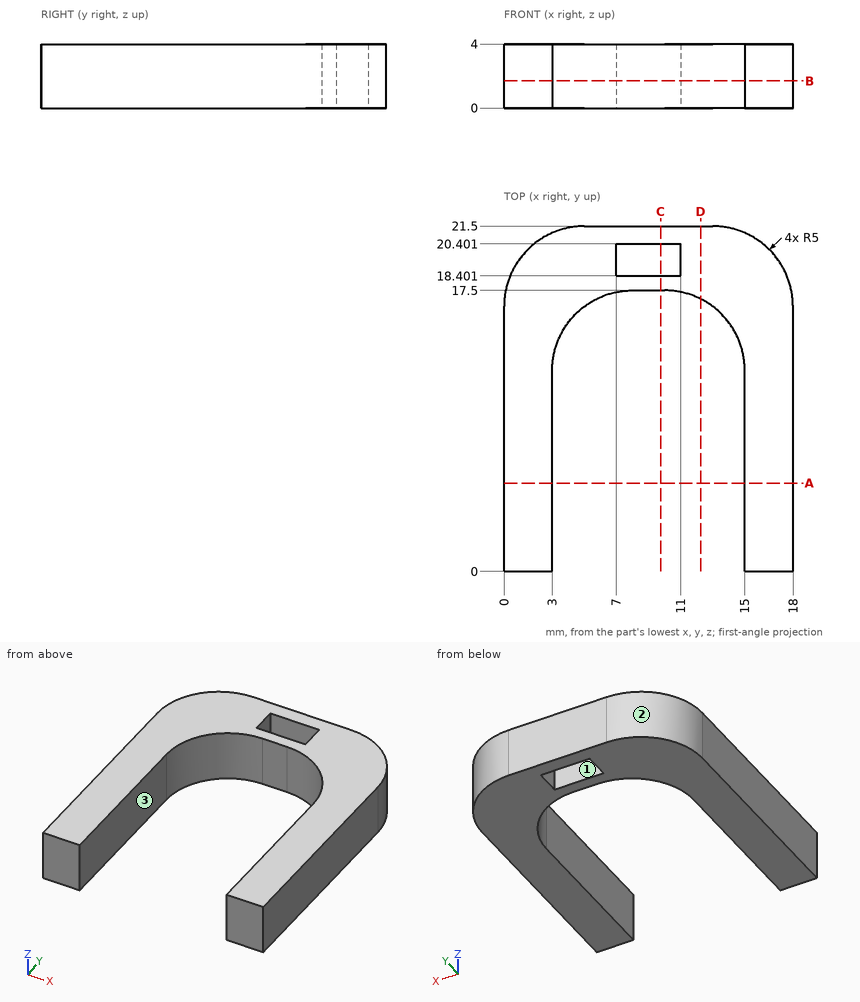
Input: dimensioned drawing with shaded views. Units: mm. Origin: part minimum x, y, z. A direction names the side the tool comes from. Round coordinates to 2 decimals unless told otherwise and drop trailing zeros. Loops run counter-clockwise (first coordinate to the right, second up) from the corner with the lowest first, then second, coordinate; pieces in that order, holes last. Notation, with made-up numbers: M 74.25,-14 L 124.25,-14 A22 ccw 124.25,6 Z; hole C 82,7 d7. An arc over 180 degrees is marked long. Answer in a Markdown table with one row per item. Add a question column.
1. Section B-B (z = 1.7). Output: boundary loops of the cut face in (x, y).
2. Section D-D (x = 12.25). Output: boundary loops of the cut face in (y, z), and give its area (3 significant figures).
3. Section A-A (y = 5.5). Output: boundary loops of the cut face in (x, z), and give its area (3 significant figures).
4. Contact query for flat-ended pins moving along their axis: pin 1 (0.6 mm diameter, centred on x = 9, z = 3, fed in from -Y); pin 2 (0.6 mm diameter, centred on y = 19.5, z = 1.5, fed in from +X); pin 3 (1 mm diameter, centred on y = 19, z = 2, fed in from -X). Output: stop coordinate, or through.
5. Ray query, probe 1 along X at (y, z) = (6.5, 1.85); probe 2 along Y at (x, z) = (9, 1.6); probe 3 along Y at (x, z) = (6, 3.3). Return the intervals inside material, ascending.
6. Set-up query: the marked faces 1, 2 and 3. Return all of +Z, -Z, +X, -X, +Y, -Y with unobstructed straight access to the full face (end or side cutting, diameter ignored); none if empty.
7. Section C-C (x = 9.75). Output: boundary loops of the cut face in (y, z).
Values follow:
| question | item | result |
|---|---|---|
| 1 | outline | M 0,0 L 3,0 L 3,12.5 A5 cw 8,17.5 L 10,17.5 A5 cw 15,12.5 L 15,0 L 18,0 L 18,16.5 A5 ccw 13,21.5 L 5,21.5 A5 ccw 0,16.5 Z; hole M 7,18.4 L 11,18.4 L 11,20.4 L 7,20.4 Z |
| 2 | outline | M 16.97,0 L 21.5,0 L 21.5,4 L 16.97,4 Z |
| 2 | area | 18.1 mm^2 |
| 3 | outline | M 0,0 L 3,0 L 3,4 L 0,4 Z; M 15,0 L 18,0 L 18,4 L 15,4 Z |
| 3 | area | 24.0 mm^2 |
| 4 | pin 1 | y = 17.5 |
| 4 | pin 2 | x = 17.21 |
| 4 | pin 3 | x = 0.42 |
| 5 | probe 1 | 0 to 3, 15 to 18 |
| 5 | probe 2 | 17.5 to 18.4, 20.4 to 21.5 |
| 5 | probe 3 | 17.08 to 21.5 |
| 6 | face 1 | +Z, -Z |
| 6 | face 2 | +Z, -Z, -X, +Y |
| 6 | face 3 | +Z, -Z, -Y |
| 7 | outline | M 17.5,0 L 18.4,0 L 18.4,4 L 17.5,4 Z; M 20.4,0 L 21.5,0 L 21.5,4 L 20.4,4 Z |
